```python
from build123d import *

# Parameters (mm, degrees)
BOSS_EXTRUDE1_DEPTH = 12.7
FILLET1_R           = 2.54


with BuildPart() as part:
    # Sketch1 → Boss-Extrude1 (new body)
    with BuildSketch(Plane(origin=(0, 0, 0), x_dir=(1, 0, 0), z_dir=(0, 1, 0))):
        Polygon((0, 0), (0, 59.69), (50.8, 59.69), (50.8, 40.64), (38.1, 40.64), (38.1, 46.99), (12.7, 46.99), (12.7, 0), align=None)
    extrude(amount=BOSS_EXTRUDE1_DEPTH)

    # Fillet1
    fillet1_edges = [part.edges().sort_by_distance(p)[0] for p in [
        (0, 6.35, 0),
        (0, 6.35, -59.69),
        (50.8, 6.35, -59.69),
        (50.8, 6.35, -40.64),
        (38.1, 6.35, -40.64),
        (38.1, 6.35, -46.99),
        (12.7, 6.35, -46.99),
        (12.7, 6.35, 0),
    ]]
    fillet(fillet1_edges, radius=FILLET1_R)


solid = part.part
```
Part model, mm, in its own coordinate system. A direction names the side the tool comes from. Round coordinates to 2 decimals unless told otherwise and drop trailing zeros. Order: outer loops, then holes, each group sorted by start corner. A loop starts at its lowest first (then second) coordinate and runs counter-clockwise, first axis right, second up. Notation, with made-up numbers: M 14,-35.5 L 34,-35.5 A21 cw 34,-16.5 Z; hole C -33,-36.5 d7. An arc over 180 degrees is marked long. Answer in a Markdown table with one row per item. Add a question column.
Q1. Cut at B-B on x = 34.5. Give the cut face in (y, z), and give its area (3 significant figures).
Q2. Cut at C-C on z = -25. Give the cut face in (x, y), and give its area (3 significant figures).
Q3. Mould opens along X. For faces 4 (the face through (26, 6, -46.99)), 5 (the face through (50.8, 6, -50)), 6 (the face through (0.724, 6.439, -0.764)) say: +X half, -X half, draft (parallel to the pull), parting line (faces both ways), or undercut.
Q4. 3-axis set-ups, long thin cutter, end or side, ignore diameter. For faces 1 (the face through (6, 6, 0)), 2 (the face through (38.864, 6.439, -41.364)), 3 (the face through (45, 6, -40.64)): which of +Z, -Z, +X, -X, +Y, -Y reach the whole face in a straight line?
Q5. Pin check, flat tips, straight feed: pin 1 (6 mm diameter, centred on x = 43.5, y = 8.5, fed in from +Z); pin 2 (4 mm diameter, centred on y = 6.5, z = -25.5, fed in from +X); pin 3 (1.5 mm diameter, centred on x = 24, y = 2, fed in from +Z). Stop position of each tip, or through.
Q6. Wall check: L1, parallel to Z at x = 42.5, y = 8.75; L2, parallel to X at y = 7, z = -36; L3, parallel to Z at x = 30.5, y = 12. Give the ranges that are in metal, low to high. Write a range as from..to.
Q7. Cut at A-A on y = 4.75. Give the cut face in (x, z).
Established:
| question | item | result |
|---|---|---|
| 1 | outline | M 0,-59.69 L 12.7,-59.69 L 12.7,-46.99 L 0,-46.99 Z |
| 1 | area | 161 mm2 |
| 2 | outline | M 0,0 L 12.7,0 L 12.7,12.7 L 0,12.7 Z |
| 2 | area | 161 mm2 |
| 3 | face 4 | undercut |
| 3 | face 5 | +X half |
| 3 | face 6 | -X half |
| 4 | face 1 | +Z, +X, -X, +Y, -Y |
| 4 | face 2 | +Z, +Y, -Y |
| 4 | face 3 | +Z, +X, +Y, -Y |
| 5 | pin 1 | stops at z = -40.64 |
| 5 | pin 2 | stops at x = 12.7 |
| 5 | pin 3 | stops at z = -46.99 |
| 6 | L1 | z = -59.69..-40.64 |
| 6 | L2 | x = 0..12.7 |
| 6 | L3 | z = -59.69..-46.99 |
| 7 | outline | M 0,-57.15 A2.54 ccw 2.54,-59.69 L 48.26,-59.69 A2.54 ccw 50.8,-57.15 L 50.8,-43.18 A2.54 ccw 48.26,-40.64 L 40.64,-40.64 A2.54 ccw 38.1,-43.18 L 38.1,-44.45 A2.54 cw 35.56,-46.99 L 15.24,-46.99 A2.54 cw 12.7,-44.45 L 12.7,-2.54 A2.54 ccw 10.16,0 L 2.54,0 A2.54 ccw 0,-2.54 Z |
